Could you check a few things on this model? Use its own coordinates, in mm. Give positions to 0.01 mm unless a question says otherwise; leave off trailing zeros. Write each loop counter-clockwise with the first axis right and the second up, starting at its lowest first coordinate (ties: lowest second). Pieces come first, ordered by that corner, then holes. Notation, with made-up numbers: (76.25, 34.25) - (131.25, 34.25) arc R26 cw to (131.25, 66.25) - close; hole circle Ø1 at (-5, -7). An arc over 180 degrees is marked (long way). Answer as CSV lines item,"result". Start each with the question number.
Q1. If I drill on line 1 along Y through (x, z) = (347.5, 2.45) (3 decimals); line 2 along X through (y, z) = (-72, 2.25); line 3 along Y through (x, z) = (85, 1.3) (3 decimals), over which ranges is the centre line in solid material (lowest first)?
Q2. Imagine slicing it at C-C on y = 168.5. List the corners of the cut face in (x, z) for me (3 decimals).
Q3. We'd pull the mould along X, two halves only. Please class faces 1 (the face through (-65.68, -568.31, 1.57)), 2 (the face through (382.79, -85, 1.61)), 3 (the face through (487.11, -148, 1.57)): pulls with the +X half, pulls with the -X half, needs draft (parallel to the pull), parting line crosses it, or undercut.
Q4. Will these pins go through, and if not, where does the flat tip stop? pin 1 Ø1.5 at (y, z) = (-347.5, 1) entering from -X; pin 2 Ø7.5 at (x, y) = (81.76, 411.05) entering from -Z.
Q5. Imagine slicing it at A-A on x = -121.5. List the corners of the cut face in (y, z) for me (3 decimals), and give its area (3 significant figures).
Q6. Imagine slicing it at D-D on y = 655. List the corners of the cut face in (x, z) for me (3 decimals), and give its area (3 significant figures).
Autodesk Inventor part; units mm, degrees
ref_plane "YZ Plane" through (0, 0, 0) normal (1, 0, 0) x (0, 1, 0)
ref_plane "XZ Plane" through (0, 0, 0) normal (0, 1, 0) x (-1, 0, 0)
ref_plane "XY Plane" through (0, 0, 0) normal (0, 0, 1) x (1, 0, 0)
sketch "Sketch1" plane through (0, 0, 0) normal (0, 0, 1) x (1, 0, 0)
  circle A0 centre (0, 0) radius 69.85 construction
  line L0 (69.85, 0) -> (34.925, -60.4919) construction
  line L1 (34.925, -60.4919) -> (-34.925, -60.4919) construction
  line L2 (-34.925, -60.4919) -> (-69.85, 0) construction
  line L3 (-69.85, 0) -> (-34.925, 60.4919) construction
  line L4 (-34.925, 60.4919) -> (34.925, 60.4919) construction
  line L5 (34.925, 60.4919) -> (69.85, 0) construction
  line L6 (69.85, 0) -> (69.85, 777.875) construction
  line L7 (0, 60.4919) -> (0, -60.4919) construction
  line L8 (-69.85, 0) -> (69.85, 0) construction
  arc A1 (69.85, 777.875) -> (-319.0875, 673.6595) centre (69.85, 0) ccw
  arc A2 (-319.0875, 673.6595) -> (-673.1, 60.4919) centre (34.925, 60.4919) ccw
  arc A3 (-673.1, 60.4919) -> (-354.0125, -492.1839) centre (-34.925, 60.4919) ccw
  arc A4 (-354.0125, -492.1839) -> (214.3125, -492.1839) centre (-69.85, 0) ccw
  arc A5 (214.3125, -492.1839) -> (463.55, -60.4919) centre (-34.925, -60.4919) ccw
  arc A6 (463.55, -60.4919) -> (458.7952, 3.175) centre (34.925, -60.4919) ccw
  line L9 (458.7952, 3.175) -> (571.5, 3.175)
  line L10 (571.5, 3.175) -> (571.5, 777.875)
  line L11 (69.85, 777.875) -> (571.5, 777.875)
  line L12 (571.5, 3.175) -> (400.325, -303.4625)
  dimension "d0" = 777.875
  dimension "d1" = 139.7
  dimension "d2" = 571.5
  dimension "d3" = 774.7
  dimension "d5" = 498.475
extrude "Extrusion1" add sketch "Sketch1" along normal blind 3.175
hole "Hole1" at (0, 0, 0) direction (0, 0, 1) diameter 784.225 end through all
ref_plane "Work Plane1" through (0, 0, 1833.3831) normal (-1, 0, 0) x (0, 0, 1)
ref_plane "Work Plane2" through (0, 0, 1833.3831) normal (0, -1, 0) x (0, 0, 1)
ref_plane "Work Plane3" through (0, 0, 1833.3831) normal (0.7071, -0.7071, 0) x (0, 0, 1)
ref_plane "Work Plane4" through (0, 0, 1833.3831) normal (-0.7071, -0.7071, 0) x (0, 0, 1)
sketch "Sketch2" plane through (0, 0, 3.175) normal (0, 0, 1) x (1, 0, 0)
  circle A0 centre (0, 0) radius 392.1125
  point P0 (411.0471, 81.7624)
  dimension "d19" = 419.1
  dimension "d20" = 81.7623
hole "Hole2" at (411.0471, 81.7624, 3.175) direction (0, 0, -1) diameter 9.525 end through all
pattern_circular "Circular Pattern1" count 16 over 360 about axis through (0, 0, 1833.3831) along (0, 0, 1) of "Hole2"
properties part number "inlet side sheet" material "Steel, Mild"
Conclusion:
1,line 1,"-380.224 to -237.502, -228.177 to -181.648, 181.648 to 228.177, 237.502 to 777.875"
1,line 2,"-659.2 to -385.45, 385.45 to 529.53"
1,line 3,"-546.822 to -414.54, -407.554 to -382.789, 382.789 to 407.554, 414.54 to 777.875"
2,outline,"(-664.813, 0) - (-354.062, 0) - (-354.062, 3.175) - (-664.813, 3.175) - close; (354.062, 0) - (571.5, 0) - (571.5, 3.175) - (354.062, 3.175) - close"
3,face 1,"parting line crosses it"
3,face 2,"undercut"
3,face 3,"pulls with the +X half"
4,pin 1,"x = -526.27"
4,pin 2,"through"
5,outline,"(-565.973, 0) - (-372.814, 0) - (-372.814, 3.175) - (-565.973, 3.175) - close; (372.814, 0) - (753.973, 0) - (753.973, 3.175) - (372.814, 3.175) - close"
5,area,"1,820 mm^2"
6,outline,"(-349.6, 0) - (571.5, 0) - (571.5, 3.175) - (-349.6, 3.175) - close"
6,area,"2,920 mm^2"
